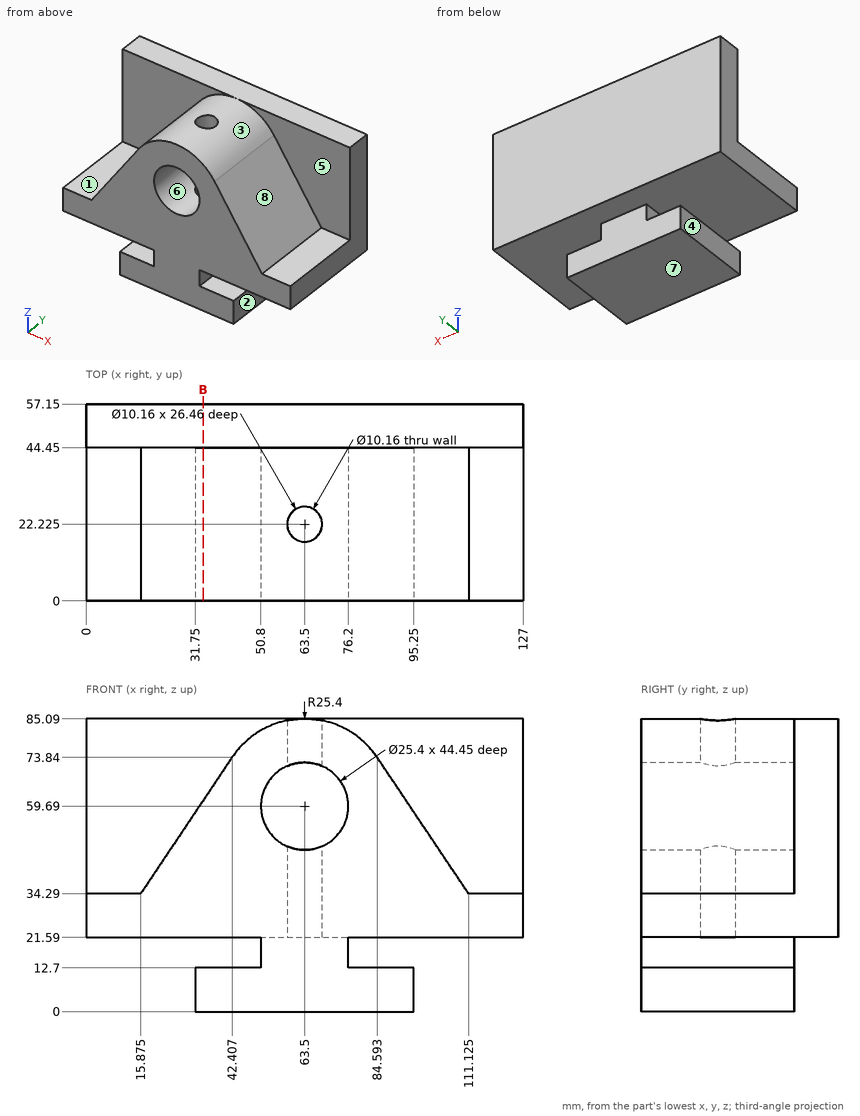
Print and shaded views of the part. All mm, measured from the part's lowest x, y and z. A direction names the side the tool comes from. Give positions to 0.01 mm unless a question says otherwise; leave off trailing zeros. Write each loop counter-clockwise with the first axis right and the second up, starting at its lowest first coordinate (ties: lowest second). Pieces come first, ordered by that corner, then holes. Notation, with made-up numbers: (-7, -18) - (-1, -18) arc R38 cw to (-1, 20) - close; hole circle Ø6 at (79, 71). An arc over 180 degrees is marked (long way). Put each result on its own line as item: value.
(1) Wall check: L1, parallel to Z at x = 63.5, y = 11.5; L2, parallel to Y at x = 63, z = 40; L3, parallel to Z at x = 121.5, y = 44.5. Give the ranges that are in metal, low to high.
Working result:
L1: 0 to 46.99, 72.39 to 85.09
L2: 0 to 17.17, 27.28 to 57.15
L3: 21.59 to 85.09
(2) Drop flat-ended pins along their axis: pin 1 Ø1 at (x, y) = (30.5, 32.5) entering from +Z (1 decimal); pin 2 Ø2 at (x, y) = (98.5, 6) entering from +Z; pin 3 Ø4.5 at (y, z) = (13, 18) entering from +X. Give the stop position or say it passes through.
Working result:
pin 1: z = 56.8
pin 2: z = 54.6
pin 3: x = 76.2
(3) Tool access for the marked faces 1, 2, 3, 4 and 5: list every direction of +Z, -Z, +X, -X, +Y, -Y with a clear straight run to the whole face (end or side of a thin tool).
Working result:
face 1: +Z, -X, -Y
face 2: -Z, +X, +Y, -Y
face 3: +Z, -Y
face 4: -Z, -X, +Y, -Y
face 5: +Z, +X, -Y
(4) Saw through at B-B (x = 34). List the corners of the cut face in (y, z), then the cut area to 3 significant figures.
Working result:
outline: (0, 0) - (44.45, 0) - (44.45, 12.7) - (0, 12.7) - close; (0, 21.59) - (57.15, 21.59) - (57.15, 85.09) - (44.45, 85.09) - (44.45, 61.31) - (0, 61.31) - close
area: 3,140 mm^2
(5) Pull direction X, two halves, no side cores. Call the marked faces 6, 7 and 8: released by +X, released by -X, zero draft, split by the parting line, or undercut.
Working result:
face 6: undercut
face 7: zero draft
face 8: released by +X
